Check sheet for the modelled part. Datum: model origin and axes. Units: mm. A direction names the side the tool comes from. Give positions to 0.01 mm unless a question says otherwise; leave off trailing zeros. Loops run counter-clockwise (first coordinate to the right, second up) from the corner with the lowest first, then second, coordinate; pieces in that order, holes last. Notation, with made-up numbers: (1, 30) -> (24, 30) arc R9 ccw to (24, 37) -> close; hole circle Ø2 at (9.5, 17.5). An arc over 180 degrees is marked (long way). Write each question's results on one line, items separated by ' | '. Start each with the question number.
1. Cross-section at B-B on x = -1.5. Record the boundary of the cut face in (y, z).
2. Cross-section at D-D on z = 12. Record the boundary of the cut face in (x, y), and give its area (3 significant figures).
3. Material ranges on L1, parallel to Z at x = 0, y = 2.2; L2, parallel to Z at x = 4.5, y = 17.25; L3, parallel to Y at x = 4.5, z = 9, recorded low to high. Write a range as from..to.
4. Cross-section at A-A on z = -25. Record the boundary of the cut face in (x, y).
5. Mould release check, pull along Y, two halves, no side actions. Record for faces 1 (the face through (-0.45, 12.17, 15.14)), 2 (the face through (-0.488, 2.972, -22.804)), 3 (the face through (6.87, 14.09, 18.23)): +Y half, -Y half, draft (parallel to the pull), parting line (faces both ways), or undercut.
6. Cross-section at C-C on y = 17.25. Record the boundary of the cut face in (x, z).
7. Tool access check on faces 4 (the face through (8, 14, 10.15)), 5 (the face through (-1, 3, 30)), 6 (the face through (-7, 5, -7)), 7 (the face through (10, 12.265, 18)). Record the directions out of +Z, -Z, +X, -X, +Y, -Y that give a thin tool (end or side, any length) a straight path to the whole face; none if there is none.
8. Gauge pin test, flat ends, axial feed: pin 1 Ø1.5 at (y, z) = (18, -9.5) entering from -X; pin 2 Ø6 at (x, y) = (9.5, 15) entering from +Z; pin 3 Ø6 at (x, z) = (0, -25) entering from +Y. Record the tip position at first contact, or that the pin passes through.
from build123d import *

# Parameters (mm, degrees)
SKETCH1_W           = 20
SKETCH1_H           = 60
SKETCH1_R           = 2.25
BOSS_EXTRUDE1_DEPTH = 5
SKETCH2_R           = 2.25
BOSS_EXTRUDE2_DEPTH = 9.85
SKETCH3_R           = 2.25
BOSS_EXTRUDE3_DEPTH = 9.85
SKETCH4_W           = 33.827008901
SKETCH4_H           = 72.568076527
CUT_EXTRUDE1_DEPTH  = 1
CUT_EXTRUDE2_DEPTH  = 61
CUT_EXTRUDE3_DEPTH  = 3.6


with BuildPart() as part:
    # Sketch1 → Boss-Extrude1 (new body)
    with BuildSketch(Plane(origin=(0, 0, 0), x_dir=(1, 0, 0), z_dir=(0, 1, 0))):
        Rectangle(SKETCH1_W, SKETCH1_H)
        with Locations((0, 25)):
            Circle(SKETCH1_R, mode=Mode.SUBTRACT)
        with Locations((0, -25)):
            Circle(SKETCH1_R, mode=Mode.SUBTRACT)
    extrude(amount=BOSS_EXTRUDE1_DEPTH)

    # Sketch2 → Boss-Extrude2 (add)
    with BuildSketch(Plane.XY.offset(20)):
        with BuildLine():
            Line((10, 9.86530346), (10, 5))
            Line((10, 5), (-6, 5))
            Line((-6, 5), (5.255684086, 19.53837663))
            ThreePointArc((5.255684086, 19.53837663), (15.386948998, 18.507420129), (10, 9.86530346))
        make_face()
        with Locations((10, 15.86530346)):
            Circle(SKETCH2_R, mode=Mode.SUBTRACT)
    extrude(amount=-BOSS_EXTRUDE2_DEPTH)

    # Sketch3 → Boss-Extrude3 (add)
    with BuildSketch(Plane(origin=(0, 0, -10), x_dir=(-1, 0, 0), z_dir=(0, 0, -1))):
        with BuildLine():
            Line((-10, 9.86530346), (-10, 5))
            Line((-10, 5), (6, 5))
            Line((6, 5), (-5.293415142, 19.586601483))
            ThreePointArc((-5.293415142, 19.586601483), (-15.40036055, 18.479898253), (-10, 9.86530346))
        make_face()
        with Locations((-10, 15.86530346)):
            Circle(SKETCH3_R, mode=Mode.SUBTRACT)
    extrude(amount=-BOSS_EXTRUDE3_DEPTH)

    # Sketch4 → Cut-Extrude1 (cut)
    with BuildSketch(Plane.XZ):
        with Locations((1.488581003, -1.778467764)):
            Rectangle(SKETCH4_W, SKETCH4_H)
    extrude(amount=-CUT_EXTRUDE1_DEPTH, mode=Mode.SUBTRACT)

    # Sketch5 → Cut-Extrude2 (cut, through all)
    with BuildSketch(Plane(origin=(0, 0, -30), x_dir=(-1, 0, 0), z_dir=(0, 0, -1))):
        Polygon((-10, 9.86530346), (-10, 1), (-8.5, 1), align=None)
    extrude(amount=-CUT_EXTRUDE2_DEPTH, mode=Mode.SUBTRACT)

    # Sketch6 → Cut-Extrude3 (cut)
    with BuildSketch(Plane.XY.offset(20)):
        Polygon((12.078460969, 12.26530346), (14.156921938, 15.86530346), (12.078460969, 19.46530346), (7.921539031, 19.46530346), (5.843078062, 15.86530346), (7.921539031, 12.26530346), align=None)
    extrude(amount=-CUT_EXTRUDE3_DEPTH, mode=Mode.SUBTRACT)


solid = part.part
Geometry says:
1) outline: (1, -30) -> (5, -30) -> (5, -26.68) -> (1, -26.68) -> close; (1, -23.32) -> (5, -23.32) -> (5, -10) -> (10.81, -10) -> (10.81, -0.15) -> (5, -0.15) -> (5, 10.15) -> (10.81, 10.15) -> (10.81, 20) -> (5, 20) -> (5, 23.32) -> (1, 23.32) -> close; (1, 26.68) -> (5, 26.68) -> (5, 30) -> (1, 30) -> close
2) outline: (-10, 1) -> (8.5, 1) -> (10, 9.87) arc R6 ccw (long way) to (5.26, 19.54) -> (-6, 5) -> (-10, 5) -> close; hole circle Ø4.5 at (10, 15.87) | area: 272 mm^2
3) L1: -30..-27.25, -22.75..22.75, 27.25..30 | L2: -10..-0.15, 10.15..20 | L3: 1..5
4) outline: (-10, 1) -> (-2.25, 1) -> (-2.25, 5) -> (-10, 5) -> close; (2.25, 1) -> (8.5, 1) -> (9.18, 5) -> (2.25, 5) -> close
5) face 1: +Y half | face 2: draft | face 3: undercut
6) outline: (3.48, -10) -> (8.23, -10) -> (8.23, -0.15) -> (3.48, -0.15) -> close; (3.48, 10.15) -> (8.23, 10.15) -> (8.23, 16.4) -> (6.64, 16.4) -> (6.64, 20) -> (3.48, 20) -> close; (11.77, -10) -> (15.84, -10) -> (15.84, -0.15) -> (11.77, -0.15) -> close; (11.77, 10.15) -> (15.84, 10.15) -> (15.84, 20) -> (13.36, 20) -> (13.36, 16.4) -> (11.77, 16.4) -> close
7) face 4: +X, -X, +Y | face 5: +Z, +X, -X, +Y, -Y | face 6: -X, +Y | face 7: +Z
8) pin 1: x = 3.48 | pin 2: z = 20 | pin 3: y = 5
